```python
from build123d import *

# Parameters (mm, degrees)
SKETCH1_W               = 130
SKETCH1_H               = 120
BOSS_EXTRUDE1_DEPTH     = 3
CUT_EXTRUDE1_START      = -4
SKETCH2_W               = 20
SKETCH2_H               = 95
CUT_EXTRUDE1_DEPTH      = 5
CUT_EXTRUDE2_START      = -4
SKETCH3_R               = 1.6
CUT_EXTRUDE2_DEPTH      = 5
SKETCH4_W               = 130
SKETCH4_H               = 82
CUT_EXTRUDE3_DEPTH      = 1
CUT_EXTRUDE3_DEPTH_BACK = 4


with BuildPart() as part:
    # Sketch1 → Boss-Extrude1 (new body)
    with BuildSketch(Plane(origin=(0, 0, 0), x_dir=(1, 0, 0), z_dir=(0, 1, 0))):
        Rectangle(SKETCH1_W, SKETCH1_H)
    extrude(amount=BOSS_EXTRUDE1_DEPTH)

    # Sketch2 → Cut-Extrude1 (cut)
    with BuildSketch(Plane(origin=(0, 3, 0), x_dir=(1, 0, 0), z_dir=(0, 1, 0)).offset(CUT_EXTRUDE1_START)):
        with Locations((-16.25, 0)):
            Rectangle(SKETCH2_W, SKETCH2_H)
    cut_extrude1 = extrude(amount=CUT_EXTRUDE1_DEPTH, mode=Mode.SUBTRACT)

    # Mirror1: Cut-Extrude1 across plane
    add(cut_extrude1.mirror(Plane(origin=(0, 0, 0), x_dir=(0, 0, 1), z_dir=(1, 0, 0))), mode=Mode.SUBTRACT)

    # Sketch3 → Cut-Extrude2 (cut)
    with BuildSketch(Plane(origin=(0, 3, 0), x_dir=(1, 0, 0), z_dir=(0, 1, 0)).offset(CUT_EXTRUDE2_START)):
        with Locations((44.5, 0)):
            Circle(SKETCH3_R)
    cut_extrude2 = extrude(amount=CUT_EXTRUDE2_DEPTH, mode=Mode.SUBTRACT)

    # Mirror2: Cut-Extrude2 across plane
    add(cut_extrude2.mirror(Plane(origin=(0, 0, 0), x_dir=(0, 0, 1), z_dir=(1, 0, 0))), mode=Mode.SUBTRACT)

    # Sketch4 → Cut-Extrude3 (cut, two sides)
    with BuildSketch(Plane(origin=(0, 3, 0), x_dir=(1, 0, 0), z_dir=(0, 1, 0))) as cut_extrude3_sk:
        with Locations((0, 19)):
            Rectangle(SKETCH4_W, SKETCH4_H)
    extrude(amount=CUT_EXTRUDE3_DEPTH, mode=Mode.SUBTRACT)
    extrude(cut_extrude3_sk.sketch, amount=-CUT_EXTRUDE3_DEPTH_BACK, mode=Mode.SUBTRACT)


solid = part.part
```
Could you check a few things on this model? Use its own coordinates, in mm. A direction names the side the tool comes from. Round coordinates to 2 decimals unless told otherwise and drop trailing zeros. Loops run counter-clockwise (first coordinate to the right, second up) from the corner with the lowest first, then second, coordinate; pieces in that order, holes last. Notation, with made-up numbers: (66, 49) -> (94, 49) arc R29 cw to (94, 71) -> close; hole circle Ø6 at (-8, 8). An arc over 180 degrees is marked (long way). Put each result on its own line as item: value.
Q1. I want a section at A-A on z = 34.5. Write out the boundary of the cut face in (x, y).
Checks:
outline: (-65, 0) -> (-26.25, 0) -> (-26.25, 3) -> (-65, 3) -> close; (-6.25, 0) -> (6.25, 0) -> (6.25, 3) -> (-6.25, 3) -> close; (26.25, 0) -> (65, 0) -> (65, 3) -> (26.25, 3) -> close
Q2. Please list where these lines run through material, in increasing order: line 1 (X direction, y = 2.45, z = 40); line 2 (Z direction, x = -24, y = 0.6). Write a range as from..to.
Checks:
line 1: -65..-26.25, -6.25..6.25, 26.25..65
line 2: 47.5..60
Q3. Thinking about a two-plate mould opening in X: for faces 1 (the flat face through (-65, 1, 41)), 2 (the flat face through (-1, 1, 60)), 3 (the flat face through (-6.25, 1, 35)), 4 (the flat face through (65, 1, 41)), which applies, pulls with the +X half, pulls with the -X half, needs draft (parallel to the pull), parting line crosses it, or undercut?
Checks:
face 1: pulls with the -X half
face 2: needs draft
face 3: undercut
face 4: pulls with the +X half
Q4. I want a section at B-B on y = 2. Write out the boundary of the cut face in (x, z).
Checks:
outline: (-65, 22) -> (-26.25, 22) -> (-26.25, 47.5) -> (-6.25, 47.5) -> (-6.25, 22) -> (6.25, 22) -> (6.25, 47.5) -> (26.25, 47.5) -> (26.25, 22) -> (65, 22) -> (65, 60) -> (-65, 60) -> close
Q5. Which directions (+Z, -Z, +X, -X, +Y, -Y) give clear straight access to the entire face, cutting with the end or side of a thin tool? Please do faces 5 (the flat face through (0, 2, 22)), 6 (the flat face through (-26.25, 1, 35)).
Checks:
face 5: -Z, +X, -X, +Y, -Y
face 6: -Z, +Y, -Y
Q6. For pin 1 Ø0.9 at (x, y) = (-15, 2) entering from -Z, with a flat end and sliding along its axis, tell me the tip position at first contact or that it passes through.
Checks:
pin 1: z = 47.5
Q7. I want a section at C-C on x = 9.5. Write out the boundary of the cut face in (y, z).
Checks:
outline: (0, 47.5) -> (3, 47.5) -> (3, 60) -> (0, 60) -> close
